```python
from build123d import *

# Parameters (mm, degrees)
ESBO_O1_R                = 5
RESSALTO_EXTRUS_O1_DEPTH = 9.5
ESBO_O2_R                = 2.25
CORTE_EXTRUS_O1_DEPTH    = 11
ESBO_O3_R                = 3
RESSALTO_EXTRUS_O2_DEPTH = 10
CORTE_EXTRUS_O2_DEPTH    = 9
FILETE1_R                = 0.5
FILETE2_R                = 0.3
CHANFRO1_SIZE            = 1


with BuildPart() as part:
    # Esboço1 → Ressalto-extrusão1 (new body)
    with BuildSketch(Plane.XY):
        with Locations((-26.183327478, 4.383756345)):
            Circle(ESBO_O1_R)
    extrude(amount=RESSALTO_EXTRUS_O1_DEPTH)

    # Esboço2 → Corte-extrusão1 (cut)
    with BuildSketch(Plane.XY.offset(9.5)):
        with Locations((-26.183327478, 4.383756345)):
            Circle(ESBO_O2_R)
    extrude(amount=-CORTE_EXTRUS_O1_DEPTH, mode=Mode.SUBTRACT)

    # Esboço3 → Ressalto-extrusão2 (add)
    with BuildSketch(Plane(origin=(0, 0, 0), x_dir=(-1, 0, 0), z_dir=(0, 0, -1))):
        with Locations(Location((26.183327478, 4.383756345, 0), (0, 0, 180))):
            Circle(ESBO_O3_R)
    extrude(amount=RESSALTO_EXTRUS_O2_DEPTH)

    # Esboço4 → Corte-extrusão2 (cut)
    with BuildSketch(Plane.XY.offset(9.5)):
        with BuildLine():
            Line((-31.183327478, 4.583756345), (-21.183327478, 4.583756345))
            ThreePointArc((-21.183327478, 4.583756345), (-20.983327478, 4.383756345), (-21.183327478, 4.183756345))
            Line((-21.183327478, 4.183756345), (-31.183327478, 4.183756345))
            ThreePointArc((-31.183327478, 4.183756345), (-31.383327478, 4.383756345), (-31.183327478, 4.583756345))
        make_face()
    extrude(amount=-CORTE_EXTRUS_O2_DEPTH, mode=Mode.SUBTRACT)

    # Filete1
    filete1_edges = [part.edges().sort_by_distance(p)[0] for p in [
        (-26.183327478, 2.133756345, 9.5),
        (-26.183327478, 6.633756345, 9.5),
    ]]
    fillet(filete1_edges, radius=FILETE1_R)

    # Filete2
    filete2_edges = [part.edges().sort_by_distance(p)[0] for p in [
        (-31.183327478, 4.383756345, 0),
    ]]
    fillet(filete2_edges, radius=FILETE2_R)

    # Chanfro1
    # the kernel refuses this chamfer: 1 mm, written as the material it adds along each edge
    with BuildSketch(Plane(origin=(-26.183327478, 4.383756345, 0), x_dir=(1, 0, 0), z_dir=(0, -1, 0))) as chanfro1_piece_1_section:
        Polygon((2.25, CHANFRO1_SIZE), (2.25 - CHANFRO1_SIZE, 0), (2.25, 0), align=None)
    chanfro1_piece_1 = revolve(axis=Axis((-26.183327478, 4.383756345, 0), (0, 0, 1)), mode=Mode.PRIVATE)
    chanfro1_piece_1 = split(chanfro1_piece_1, bisect_by=Plane(origin=(-24.32601133, 4.383756345, 0.5), z_dir=(0, 0, -1)), keep=Keep.TOP, mode=Mode.PRIVATE)
    add(chanfro1_piece_1)
    with BuildSketch(Plane(origin=(-26.183327478, 4.383756345, 0), x_dir=(1, 0, 0), z_dir=(0, -1, 0))) as chanfro1_piece_2_section:
        Polygon((2.25, CHANFRO1_SIZE), (2.25 - CHANFRO1_SIZE, 0), (2.25, 0), align=None)
    chanfro1_piece_2 = revolve(axis=Axis((-26.183327478, 4.383756345, 0), (0, 0, 1)), mode=Mode.PRIVATE)
    chanfro1_piece_2 = split(chanfro1_piece_2, bisect_by=Plane(origin=(-26.183327478, 4.583756345, 0.743524391), z_dir=(0, 1, 0)), keep=Keep.TOP, mode=Mode.PRIVATE)
    add(chanfro1_piece_2)
    with BuildSketch(Plane(origin=(-26.183327478, 4.383756345, 0), x_dir=(1, 0, 0), z_dir=(0, -1, 0))) as chanfro1_piece_3_section:
        Polygon((2.25, CHANFRO1_SIZE), (2.25 - CHANFRO1_SIZE, 0), (2.25, 0), align=None)
    chanfro1_piece_3 = revolve(axis=Axis((-26.183327478, 4.383756345, 0), (0, 0, 1)), mode=Mode.PRIVATE)
    chanfro1_piece_3 = split(chanfro1_piece_3, bisect_by=Plane(origin=(-26.183327478, 4.183756345, 0.743524391), z_dir=(0, -1, 0)), keep=Keep.TOP, mode=Mode.PRIVATE)
    add(chanfro1_piece_3)


solid = part.part
```
Verification items for the finished model (mm, model axes). A direction names the side the tool comes from. Coordinates: 2 decimals unless noted, no trailing zeros. Order: outer loops, then holes, each group sorted by start corner. A loop starts at its lowest first (then second) coordinate and runs counter-clockwise, first axis right, second up. Notation, with made-up numbers: (-22.75, 43.5) -> (29.25, 43.5) arc R24 cw to (29.25, 62.5) -> close; hole circle Ø3 at (-31, 39). An arc over 180 degrees is marked (long way). Put each result on its own line as item: value. Start each with the question number.
1) Material ranges on L1, parallel to Z at x = -26.25, y = 1.25; L2, parallel to Z at x = -25.75, y = 4.5; L3, parallel to X at y = 4.5, z = -1, recorded low to high.
2) Tool access check on faces 5 (the flat face through (-26, 1, 0)), 6 (the flat face through (-26, 4, 0)), 7 (the flat face through (-22, 4.184, 5)). Record the directions out of +Z, -Z, +X, -X, +Y, -Y that give a thin tool (end or side, any length) a straight path to the whole face; none if there is none.
3) Release check for a two-part mould opening along X. For faces 1 (the flat face through (-30, 4.184, 5)), 2 (the conical face through (-24.84, 4.81, 0.16)), 3 (the cylindrical face through (-26.137, 6.633, 5.056)), 4 (the cylindrical face through (-23.4, 5.5, -4.9)) record: pulls with the +X half, pulls with the -X half, needs draft (parallel to the pull), parting line crosses it, or undercut.
4) Cross-section at B-B (z = -7.25). Enter the section's corners in (x, y), plus the area to 3 significant figures.
5) Cross-section at A-A (z = 7.5). Enter the section's corners in (x, y).
6) Go/stop test with flat-tipped pins: pin 1 (2.5 mm diameter, centred on x = -23, z = 4.5, fed in from -Y); pin 2 (3.5 mm diameter, centred on x = -22, z = 7, fed in from +Y); pin 3 (1 mm diameter, centred on x = -23, z = 5.5, fed in from -Y); pin 4 (5 mm diameter, centred on x = -22.5, y = 2, fed in from -Z). Record where each tip stops, or that it passes through.
Geometry check:
1. L1: z = 0 to 9.5
1. L2: z = -10 to 0
1. L3: x = -29.18 to -23.19
2. face 5: -Z
2. face 6: +Z
2. face 7: +Z, +X, -X
3. face 1: needs draft
3. face 2: undercut
3. face 3: undercut
3. face 4: parting line crosses it
4. outline: circle Ø6 at (-26.18, 4.38)
4. area: 28.3 mm^2
5. outline: (-31.18, 4.18) arc R5 ccw to (-21.19, 4.18) -> (-23.94, 4.18) arc R2.25 cw to (-28.42, 4.18) -> close; (-31.18, 4.58) -> (-28.42, 4.58) arc R2.25 cw to (-23.94, 4.58) -> (-21.19, 4.58) arc R5 ccw to start
6. pin 1: stops at y = -0.23
6. pin 2: stops at y = 8.75
6. pin 3: stops at y = 0.16
6. pin 4: stops at z = -10
